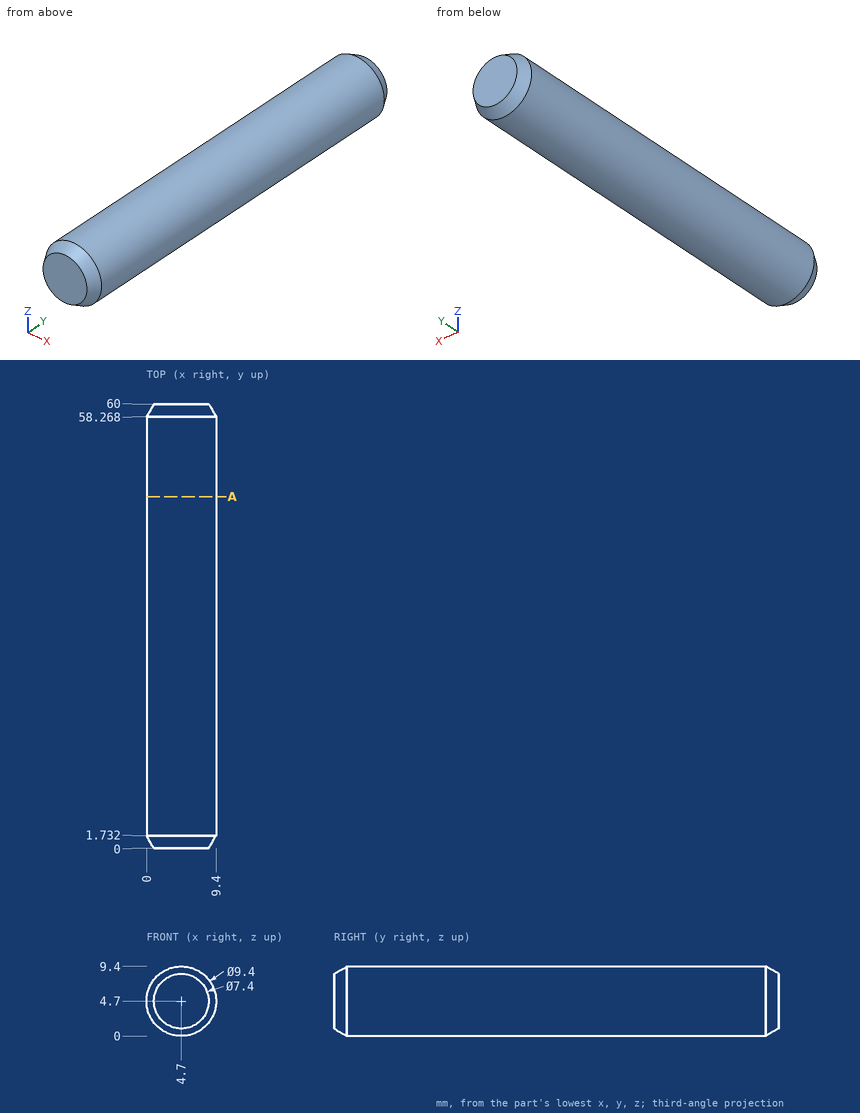
Geometry check sheet. Reference: drawing and pictorial views, mm from the part's lowest x, y, z. Coordinates: 2 decimals unless noted, no trailing zeros. Order: outer loops, then holes, each group sorted by start corner. A loop starts at its lowest first (then second) coordinate and runs counter-clockwise, first axis right, second up. Notation, with made-up numbers: (22.5, 86) -> (45.5, 86) arc R24 cw to (45.5, 96) -> close; hole circle Ø5 at (63, -35). An arc over 180 degrees is marked (long way). Put each result on its own line as item: value. Start each with the question number.
1) Material ranges on L1, parallel to Z at x = 5, y = 11.5; L2, parallel to X at y = 46, z = 6.75; L3, parallel to X at y = 26, z = 6, recorded low to high.
2) Cross-section at A-A (y = 47.5). Enter the section's corners in (x, z).
3) Go/stop test with flat-tipped pins: pin 1 (2 mm diameter, centred on x = 1.5, z = 1, fed in from +Y); pin 2 (4 mm diameter, centred on y = 21, z = 7.5, fed in from -X); pin 3 (1 mm diameter, centred on x = 1, z = 7.5, fed in from +Y). Record where each tip stops, or that it passes through.
Geometry check:
1. L1: z = 0.01 to 9.39
1. L2: x = 0.47 to 8.93
1. L3: x = 0.18 to 9.22
2. outline: circle Ø9.4 at (4.7, 4.7)
3. pin 1: stops at y = 59.67
3. pin 2: stops at x = 0.07
3. pin 3: stops at y = 59.24
